Could you check a few things on this model? Use its own coordinates, in mm. Face numbers are marked on the shaded views. A direction names the side the tool comes from. Round coordinates to 2 decimals unless told otherwise and drop trailing zeros. Loops run counter-clockwise (first coordinate to the right, second up) from the corner with the lowest first, then second, coordinate; pieces in that order, holes last. Notation, with made-up numbers: (10, -17) -> (40, -17) arc R18 ccw to (40, 3) -> close; hole circle Ø6 at (-27, 68.25). An arc over 180 degrees is marked (long way). Use CSV: the item, a comma, the result in double quotes. Start each with the question number.
```python
from build123d import *

# Parameters (mm, degrees)
F0_R      = 11.5
F1_DEPTH  = 23
F2_R      = 10
F3_DEPTH  = 4
F4_W      = 0.1
F4_H      = 2.3364797575
F5_DEPTH  = 5
F6_R      = 1
F7_DEPTH  = 25
F8_R      = 1.1
F10_R     = 2.5
F11_DEPTH = 33
F12_R     = 11.1951487388
F12_R_2   = 7.7112913891
F13_DEPTH = 0.01
F14_R     = 2.5
F15_DEPTH = 0.5
F16_R     = 3.5
F17_DEPTH = 4
F18_R     = 2.5
F19_DEPTH = 1


with BuildPart() as f1:
    # F0 (on Front) → F1 (new body)
    with BuildSketch(Plane.XZ):
        Circle(F0_R)
    extrude(amount=F1_DEPTH)

    # F2 (on face) → F3 (join)
    with BuildSketch(Plane(origin=(0, 0, 0), x_dir=(-1, 0, 0), z_dir=(0, 1, 0))):
        Circle(F2_R)
    extrude(amount=F3_DEPTH)

    # F4 (on face) → F5 (join)
    with BuildSketch(Plane.XZ.offset(23)):
        with Locations((-8.0499843252, 0.0158365793)):
            Rectangle(F4_W, F4_H)
    extrude(amount=F5_DEPTH)

    # F6 (on face) → F7 (cut)
    with BuildSketch(Plane.YZ.offset(-7.9999843252)):
        with Locations((-25.5, 0)):
            Circle(F6_R)
    extrude(amount=-F7_DEPTH, mode=Mode.SUBTRACT)

    # F8
    f8_edges = [f1.edges().sort_by_distance(p)[0] for p in [
        (-8.049984, -28, -1.152403),
        (-8.049984, -28, 1.184076),
    ]]
    fillet(f8_edges, radius=F8_R)

    # F9: F1 across plane


with BuildPart() as f1_1:
    add(f1.part)
    add(f1.part.mirror(Plane.YZ))

    # F10 (on face) → F11 (join)
    with BuildSketch(Plane.XZ.offset(23)):
        Circle(F10_R)
    extrude(amount=-F11_DEPTH)

    # F12 (on face) → F13 (join)
    with BuildSketch(Plane.XZ.offset(23)):
        Circle(F12_R)
        Circle(F12_R_2, mode=Mode.SUBTRACT)
    extrude(amount=F13_DEPTH)

    # F14 (on face) → F15 (join)
    with BuildSketch(Plane.XZ.offset(23)):
        Circle(F14_R)
    extrude(amount=F15_DEPTH)

    # F16 (on face) → F17 (join)
    with BuildSketch(Plane(origin=(0, 10, 0), x_dir=(-1, 0, 0), z_dir=(0, 1, 0))):
        Circle(F16_R)
    extrude(amount=F17_DEPTH)

    # F18 (on face) → F19 (cut)
    with BuildSketch(Plane(origin=(0, 14, 0), x_dir=(-1, 0, 0), z_dir=(0, 1, 0))):
        Circle(F18_R)
    extrude(amount=-F19_DEPTH, mode=Mode.SUBTRACT)


solid = f1_1.part
```
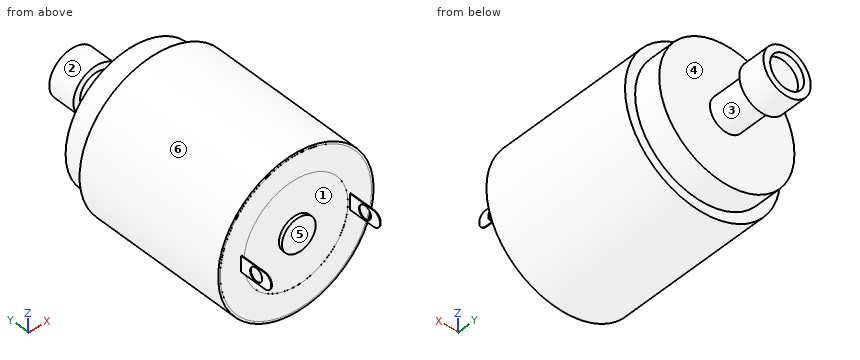
1. Will these pins go through, and if not, where does the flat tip stop? pin 1 (3 mm diameter, centred on x = 2.5, y = -23, fed in from -Z); pin 2 (4 mm diameter, centred on y = 2.5, z = -6, fed in from -X); pin 3 (8 mm diameter, centred on x = -7.5, z = -5.5, fed in from -Y); pin 4 (1.8 mm diameter, centred on y = -25.5, z = 0, fed in from +X).
2. If I drill on L1, parallel to Z at x = 0, y = 13.7; L2, parallel to Y at x = -6.75, z = 8.25; L3, parallel to Y at x = 1.75, z = -1, over which ranges is the centre line in solid material (lowest first)?
3. We'd pull the mould along X, two halves only. Please class the marked faces 4, 5 and 6: pulls with the +X half, pulls with the -X half, needs draft (parallel to the pull), parting line crosses it, or undercut.
4. Suppose I cut it at A-A (y = -25.5). List the corners of the cut face in (x, z) for me.
5. Suppose I cut it at D-D (y = 6). List the corners of the cut face in (x, z) for me, then the cut area to 3 significant figures.
6. For the marked faces 1, 2 and 3, which set-ups out of +Z, -Z, +X, -X, +Y, -Y let a thin tool reach every point of the face, with its end or its side?
Geometry check:
1,pin 1,"stops at z = -11.46"
1,pin 2,"stops at x = -9.17"
1,pin 3,"stops at y = -23.01"
1,pin 4,"passes through"
2,L1,"z = -3.5 to -2.5, 2.5 to 3.5"
2,L2,"y = -23.01 to 0"
2,L3,"y = -23.5 to 13"
3,face 4,"needs draft"
3,face 5,"undercut"
3,face 6,"parting line crosses it"
4,outline,"(-8.1, -1.15) -> (-8, -1.15) -> (-8, -1) -> (-8.1, -1) -> close; (-8.1, 1) -> (-8, 1) -> (-8, 1.18) -> (-8.1, 1.18) -> close; (8, -1.15) -> (8.1, -1.15) -> (8.1, -1) -> (8, -1) -> close; (8, 1) -> (8.1, 1) -> (8.1, 1.18) -> (8, 1.18) -> close"
5,outline,"circle Ø5 at (0, 0)"
5,area,"19.6 mm²"
6,face 1,"-Y"
6,face 2,"+Y"
6,face 3,"none"
